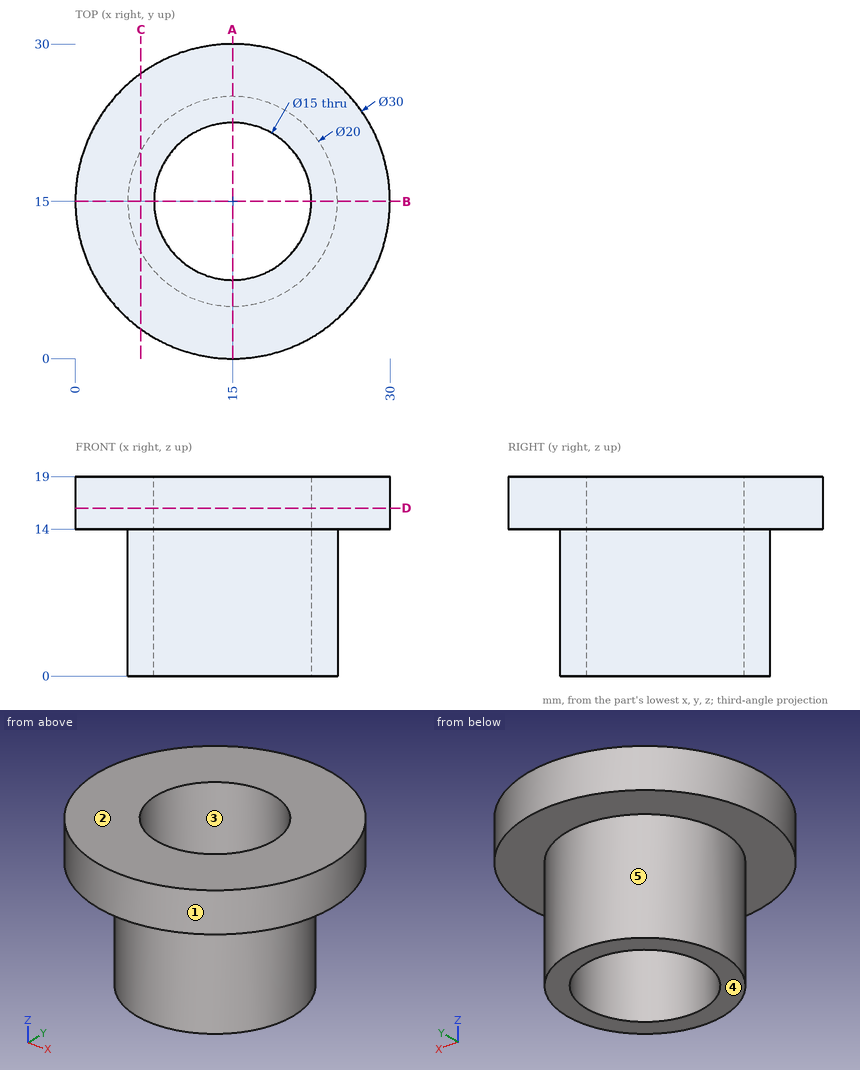
Geometry: see drawing. Coordinates: mm, zero at the bounding-box minimum. A direction names the side the tool comes from. Give positions to 0.01 mm unless a question says otherwise; leave off trailing zeros. Write each loop counter-clockwise with the first axis right and the second up, starting at its lowest first coordinate (ties: lowest second). Pieces come first, ordered by that corner, then holes. Notation, with made-up numbers: (70.5, -30.5) - (93.5, -30.5) arc R16 cw to (93.5, 0.5) - close; hole circle Ø1 at (83, 71). An arc over 180 degrees is marked (long way). Return JSON: item names as keys, results as strings. Group by question number.
1) Line query: line 1 (Y direction, x = 15, z = 6.5); line 2 (Z direction, x = 23.5, y = 7); line 3 (Y direction, x = 17.25, z = 5.5). Output: solid intervals per line, ascending.
2) Section C-C on x = 6.25. Return the cut outline in (y, z).
3) Set-up query: the marked faces 4 and 5. Return all of +Z, -Z, +X, -X, +Y, -Y with unobstructed straight access to the full face (end or side cutting, diameter ignored); none if empty.
4) Mould query, pull axis Y, two halves, no side actions, for the marked faces 1, 2 and 3. Classes: released by +Y, released by -Y, zero draft, split by the parting line, or undercut.
5) Section D-D on z = 16. Return the cut outline in (x, y).
6) First-contact query: P1, Ø2, axis at x = 27, y = 5, coming from the +Z side; P2, Ø3, axis at y = 19, z = 17, coming from the +X side; P3, Ø1.5, axis at y = 17.5, z = 5.5, coming from the -X side; P4, Ø6, axis at x = 23.5, z = 7, coming from the +Y side. Flat tips, straight axial feed; report the tip coordinate or a pass-through.
7) Section A-A on x = 15. Return the cut outline in (y, z), plus the area to 3 significant figures.
Filled in:
{
 "1": {"line 1": "y = 5 to 7.5, 22.5 to 25", "line 2": "z = 14 to 19", "line 3": "y = 5.26 to 7.85, 22.15 to 24.74"},
 "2": {"outline": "(2.82, 14) - (10.16, 14) - (10.16, 0) - (19.84, 0) - (19.84, 14) - (27.18, 14) - (27.18, 19) - (2.82, 19) - close"},
 "3": {"face 4": "-Z, +X, -X, +Y, -Y", "face 5": "-Z"},
 "4": {"face 1": "split by the parting line", "face 2": "zero draft", "face 3": "undercut"},
 "5": {"outline": "circle Ø30 at (15, 15); hole circle Ø15 at (15, 15)"},
 "6": {"P1": "stops at z = 19", "P2": "stops at x = 29.79", "P3": "stops at x = 5.15", "P4": "stops at y = 23.35"},
 "7": {"outline": "(0, 14) - (5, 14) - (5, 0) - (7.5, 0) - (7.5, 19) - (0, 19) - close; (22.5, 0) - (25, 0) - (25, 14) - (30, 14) - (30, 19) - (22.5, 19) - close", "area": "145 mm^2"}
}
